Part model, mm, in its own coordinate system. A direction names the side the tool comes from. Give positions to 0.01 mm unless a question says otherwise; leave off trailing zeros. Order: outer loops, then holes, each group sorted by start corner. A loop starts at its lowest first (then second) coordinate and runs counter-clockwise, first axis right, second up. Notation, with made-up numbers: M -4,79 L 8,79 A25 cw 8,106 Z; hole C 13.5,76 d9. An arc over 180 degrees is marked long. Return JSON: item names as keys, results as strings.
from build123d import *

# Parameters (mm, degrees)
F1_R     = 50
F1_W     = 60
F1_H     = 60
F2_DEPTH = 10
F3_R     = 2.5
F4_DEPTH = 145
F6_COUNT = 2
F6_ANGLE = 90


with BuildPart() as f2:
    # F1 (on Top) → F2 (new body)
    with BuildSketch(Plane.XY):
        Circle(F1_R)
        Rectangle(F1_W, F1_H, mode=Mode.SUBTRACT)
    extrude(amount=F2_DEPTH)


with BuildPart() as f4:
    # F3 (on face) → F4 (new body, symmetric)
    with BuildSketch(Plane.XZ.offset(-30)):
        with Locations((-24, 5)):
            Circle(F3_R)
    extrude(amount=F4_DEPTH, both=True)


with BuildPart() as f4b:
    # F3 (on face) → F4, piece 2 (new body, symmetric)
    with BuildSketch(Plane.XZ.offset(-30)):
        with Locations((24, 5)):
            Circle(F3_R)
    extrude(amount=F4_DEPTH, both=True)


with BuildPart() as f6_1:
    # F6: instance of F4
    add(f4.part.rotate(Axis((0, 0, 22.8316206485), (0, 0, 1)), 1 * F6_ANGLE / (F6_COUNT - 1)))


with BuildPart() as f6_2:
    # F6: instance of F4b
    add(f4b.part.rotate(Axis((0, 0, 22.8316206485), (0, 0, 1)), 1 * F6_ANGLE / (F6_COUNT - 1)))


with BuildPart() as f2_1:
    add(f2.part)

    # F7: cut F4, F6_2, F4b, F6_1
    add(f4.part, mode=Mode.SUBTRACT)
    add(f6_2.part, mode=Mode.SUBTRACT)
    add(f4b.part, mode=Mode.SUBTRACT)
    add(f6_1.part, mode=Mode.SUBTRACT)


solid = f2_1.part
Q1. Two-plate mould, pull along Z, no slides. Class faces 3 (the cylindrical face through (37.677, -21.615, 5.751)), 4 (the flat face through (0, -30, 5)), 5 (the flat face through (-1, -33, 0)): +Z half, -Z half, draft (parallel to the pull), parting line (faces both ways), or undercut.
Established:
{"face 3": "undercut", "face 4": "draft", "face 5": "-Z half"}
Q2. Pin check, flat tips, straight feed: pin 1 (3 mm diameter, centred on y = 6.5, z = 6, fed in from -X); pin 2 (6 mm diameter, centred on x = 25, y = -10, fed in from +Z); pin 3 (2 mm diameter, centred on y = -21.5, z = 7, fed in from +X); pin 4 (4 mm diameter, centred on x = -3.5, z = 3, fed in from +Y). Stop position of each tip, or through.
Established:
{"pin 1": "stops at x = -49.75", "pin 2": "passes through", "pin 3": "stops at x = 45.6", "pin 4": "stops at y = 49.98"}
Q3. Band-saw the part on C-C (y = 23.5). Give the cut face in (x, z), then the cut area to 3 significant figures.
Established:
{"outline": "M -44.13,0 L -30,0 L -30,2.55 L -44.13,2.55 Z; M -44.13,7.45 L -30,7.45 L -30,10 L -44.13,10 Z; M 30,0 L 44.13,0 L 44.13,2.55 L 30,2.55 Z; M 30,7.45 L 44.13,7.45 L 44.13,10 L 30,10 Z", "area": "144 mm²"}
Q4. Band-saw the part on A-A (y = 0). Give the cut face in (x, z), then the cut area to 3 significant figures.
Established:
{"outline": "M -50,0 L -30,0 L -30,10 L -50,10 Z; M 30,0 L 50,0 L 50,10 L 30,10 Z", "area": "400 mm²"}
Q5. 3-axis set-ups, long thin cutter, end or side, ignore diameter. For faces 1 (the flat face through (0, 30, 5)), 2 (the cylindrical face through (37.7, 21.5, 5.1)): which of +Z, -Z, +X, -X, +Y, -Y reach the whole face in a straight line?
Established:
{"face 1": "+Z, -Z", "face 2": "+X, -X"}
Q6. Band-saw the part on B-B (x = 18). Give the cut face in (y, z), then the cut area to 3 significant figures.
Established:
{"outline": "M -46.65,0 L -30,0 L -30,10 L -46.65,10 Z; M 30,0 L 46.65,0 L 46.65,10 L 30,10 Z", "area": "333 mm²"}
Q7. Band-saw the part on D-D (x = -34). Give the cut face in (y, z).
Established:
{"outline": "M -36.66,0 L 36.66,0 L 36.66,10 L -36.66,10 Z; hole C -24,5 d5; hole C 24,5 d5"}
Q8. Probe line 1 along Z through (x, y) = (-40.25, 24); line 2 along Y through (x, z) = (31, 4); line 3 along Y through (x, z) = (-36, 2.75). List the from-to ranges inside material, lowest first.
Established:
{"line 1": "z = 0 to 2.5, 7.5 to 10", "line 2": "y = -39.23 to -26.29, -21.71 to 21.71, 26.29 to 39.23", "line 3": "y = -34.7 to -25.09, -22.91 to 22.91, 25.09 to 34.7"}
